Geometry check sheet. Reference: the model listing, model coordinates, mm. Face numbers are marked on the shaded views. A direction names the side the tool comes from. Round coordinates to 2 decimals unless told otherwise and drop trailing zeros. Order: outer loops, then holes, each group sorted by start corner. A loop starts at its lowest first (then second) coordinate and runs counter-clockwise, first axis right, second up. Notation, with made-up numbers: (28, 75.25) - (58, 75.25) arc R16 ccw to (58, 99.25) - close; hole circle Ø6 at (27.25, -2). An arc over 180 degrees is marked (long way). Use a Markdown table: item, result. Add a question column.
(1) Mould release check, pull along X, two halves, no side actions. Record for the marked faces 1, 2, 3 and 4: released by +X, released by -X, zero draft, split by the parting line, or undercut.
(2) Section check D-D on y = 14. Record the boundary of the cut face in (x, z).
(3) Section check A-A on x = -17. Record the boundary of the cut face in (y, z).
(4) Thickness scan on line 1 along Y through (x, z) = (-4.6, 40) (3 decimals); line 2 along Y through (x, z) = (-22, 0); line 3 along X through (y, z) = (42.5, 23.5). Record the ranges inside material, lowest first. Write a range as [from, to].
(5) Access from +Z, -Z, +X, -X, +Y, -Y to the whole of each face (thin tool, end or side, straight path). Record for the marked faces 5, 6 and 7.
(6) Section check B-B on x = -2. Record the boundary of the cut face in (y, z) (3 decimals).
(7) Gauge pin test, flat ends, axial feed: P1, Ø2.5, axis at y = 50.125, z = 40, coming from the -X side; P2, Ø3, axis at x = -13, z = 14.5, coming from the +Y side; P3, Ø8, axis at y = 10.5, z = 38, coming from the +X side; P4, Ø3.5, axis at x = -4.5, z = 35.5, coming from the -Y side (3 decimals). Record the tip position at first contact, or that the pin passes through.
(8) Section check C-C on z = 7.5. Record the boundary of the cut face in (x, y), then the cut area to 3 significant figures.
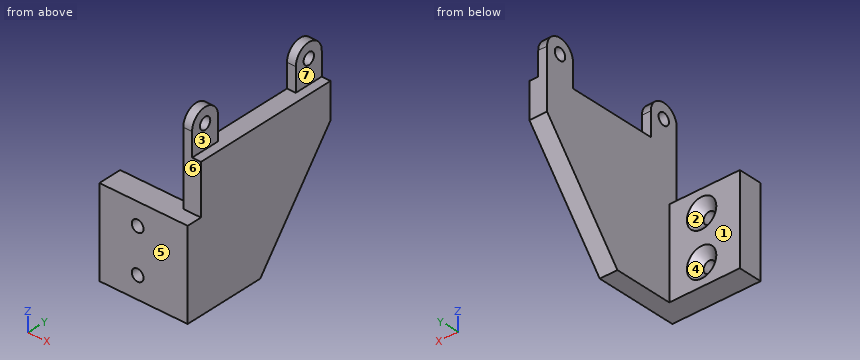
```python
from build123d import *

# Parameters (mm, degrees)
SKETCH_1_W          = 30
SKETCH_1_H          = 30
SKETCH_1_R          = 2
EXTRUDE_1_DEPTH     = 8
SKETCH_3_R          = 2
EXTRUDE_2_DEPTH     = 6
CHAMFER_1_SIZE      = 3
CUT_EXTRUDE_START   = -6
SKETCH_4_W          = 13
SKETCH_4_H          = 50
CUT_EXTRUDE_1_DEPTH = 3


with BuildPart() as part:
    # 草图1 → 凸台-拉伸1 (new body)
    with BuildSketch(Plane(origin=(0, 0, 0), x_dir=(1, 0, 0), z_dir=(0, 1, 0))):
        with Locations((-15, 0)):
            Rectangle(SKETCH_1_W, SKETCH_1_H)
        with Locations(Location((-17, 7.5, 0), (0, 0, 90))):
            Circle(SKETCH_1_R, mode=Mode.SUBTRACT)
        with Locations(Location((-17, -7.5, 0), (0, 0, 270))):
            Circle(SKETCH_1_R, mode=Mode.SUBTRACT)
    extrude(amount=EXTRUDE_1_DEPTH)

    # 草图3 → 凸台-拉伸2 (add)
    with BuildSketch(Plane(origin=(0, 0, 0), x_dir=(0, 0, -1), z_dir=(1, 0, 0))):
        with BuildLine():
            Line((-15, 8), (-15, 5.125))
            Line((-15, 5.125), (-40, 5.125))
            ThreePointArc((-40, 5.125), (-45, 10.125), (-40, 15.125))
            Line((-40, 15.125), (-32, 15.125))
            Line((-32, 15.125), (-32, 45.125))
            Line((-32, 45.125), (-40, 45.125))
            ThreePointArc((-40, 45.125), (-45, 50.125), (-40, 55.125))
            Line((-40, 55.125), (-20, 55.125))
            Line((-20, 55.125), (15, 28))
            Line((15, 28), (15, 8))
            Line((15, 8), (-15, 8))
        make_face()
        with Locations((-40, 10.125)):
            Circle(SKETCH_3_R, mode=Mode.SUBTRACT)
        with Locations((-40, 50.125)):
            Circle(SKETCH_3_R, mode=Mode.SUBTRACT)
    extrude(amount=-EXTRUDE_2_DEPTH)

    # 倒角1
    chamfer_1_edges = [part.edges().sort_by_distance(p)[0] for p in [
        (-17, 8, -5.5),
        (-17, 8, 5.5),
    ]]
    chamfer(chamfer_1_edges, length=CHAMFER_1_SIZE)

    # 草图4 → 切除-拉伸1 (cut)
    with BuildSketch(Plane.ZY.offset(6).offset(CUT_EXTRUDE_START)):
        with Locations((38.5, 30.125)):
            Rectangle(SKETCH_4_W, SKETCH_4_H)
    extrude(amount=CUT_EXTRUDE_1_DEPTH, mode=Mode.SUBTRACT)


solid = part.part
```
Check sheet entries:
| question | item | result |
|---|---|---|
| 1 | face 1 | zero draft |
| 1 | face 2 | undercut |
| 1 | face 3 | released by +X |
| 1 | face 4 | undercut |
| 2 | outline | (-6, -15) - (0, -15) - (0, 32) - (-3, 32) - (-3, 43.16) - (-6, 43.16) - close |
| 3 | outline | (0, -15) - (8, -15) - (8, -12.5) - (5, -9.5) - (0, -9.5) - close; (0, -5.5) - (5, -5.5) - (8, -2.5) - (8, 2.5) - (5, 5.5) - (0, 5.5) - close; (0, 9.5) - (5, 9.5) - (8, 12.5) - (8, 15) - (0, 15) - close |
| 4 | line 1 | y = [5.125, 8.125], [12.125, 15.125], [45.125, 48.125], [52.125, 55.125] |
| 4 | line 2 | y = [0, 8] |
| 4 | line 3 | x = [-6, 0] |
| 5 | face 5 | +Z, -Z, +X, -X, -Y |
| 5 | face 6 | +Z, +X, -X, -Y |
| 5 | face 7 | +Z, +X, +Y, -Y |
| 6 | outline | (0, -15) - (28, -15) - (55.125, 20) - (55.125, 32) - (5.125, 32) - (5.125, 15) - (0, 15) - close |
| 7 | P1 | passes through |
| 7 | P2 | stops at y = 8 |
| 7 | P3 | stops at x = -3 |
| 7 | P4 | stops at y = 5.125 |
| 8 | outline | (-30, 0) - (-19, 0) - (-19, 5) - (-22, 8) - (-30, 8) - close; (-15, 0) - (0, 0) - (0, 45.44) - (-6, 45.44) - (-6, 8) - (-12, 8) - (-15, 5) - close |
| 8 | area | 424 mm2 |
